Can you work these out from the model? Positions are in its coordinate system, mm. A direction names the side the tool comes from. Give positions to 0.01 mm unless a question says otherwise; leave off trailing zeros. Write each loop counter-clockwise with the first axis right and the second up, starting at its lowest first coordinate (ties: lowest second). Pieces come first, ordered by that corner, then holes.
1. Suppose I cut it at C-C (x = 5). Please give me the cut outline in (y, z), and give its area (3 significant figures).
2. Thinking about a two-plate mould opening in X: for faces 4 (the flat face through (48, -17.145, 3)), 5 (the cylindrical face through (-1.1, -74.92, 2.66)), 6 (the cylindrical face through (7.704, -24.063, 2.661)), which applies, pulls with the +X half, pulls with the -X half, needs draft (parallel to the pull), parting line crosses it, or undercut?
3. Suppose I cut it at D-D (y = -25.4). Give the number of separate pieces and of enclosed holes in the cut face, and give its area (3 significant figures).
4. Suppose I cut it at B-B (x = -46.99). Please give me the cut outline in (y, z) (1 decimal), and give its area (3 significant figures).
5. On a 3-axis mill with a long thin cutter (end or side, diameter ignored), from which of +Z, -Z, +X, -X, +Y, -Y can I reach the whole of each face in a straight line? I mean faces 1 (the cylindrical face through (0.41, -22.25, 2.74)), 2 (the cylindrical face through (-9.535, -20.621, 2.661)), 3 (the flat face through (54.55, -27, 3)). Say none if no direction works.
6. Suppose I cut it at A-A (y = -39.5). Please give me the cut outline in (x, z), and give its area (3 significant figures).
7. If I drill on probe 1 along X at (y, z) = (-28, 3.85); probe 2 along X at (y, z) = (-37.5, 1.35); probe 3 along X at (y, z) = (-39, 1.1), over which ranges is the centre line in solid material (lowest first)?
8. I'm going to push flat-ended pins straight in: pin 1 (5 mm diameter, centred on x = 0, y = -25.4, fed in from +Z); pin 2 (1.5 mm diameter, centred on x = 11.5, z = 2, fed in from +Y); pin 3 (1 mm diameter, centred on y = -51.5, z = 2, fed in from +X); pin 4 (1.6 mm diameter, centred on x = 34.5, z = 3, fed in from +Y) (3 decimals). Where does each tip first touch, or does it pass through?
```python
from build123d import *

# Parameters (mm, degrees)
SKETCH1_R                 = 1.651
BOSS_EXTRUDE2_DEPTH       = 5.3975
SKETCH2_R                 = 1.143
CUT_EXTRUDE1_DEPTH        = 6.3975
SKETCH3_R                 = 12.1285
CUT_EXTRUDE2_DEPTH        = 6.3975
SKETCH4_W                 = 28.562713242
SKETCH4_H                 = 11.677503754
BOSS_EXTRUDE3_DEPTH       = 5.3975
SKETCH5_W                 = 216.7214489
SKETCH5_H                 = 130.569220634
CUT_EXTRUDE4_DEPTH        = 6.3975
SKETCH7_R                 = 2
CUT_EXTRUDE5_DEPTH        = 23.368
SKETCH11_W                = 11.43
SKETCH11_H                = 10.16
CUT_EXTRUDE9_DEPTH        = 6.3975
SKETCH67_R                = 1.651
CUT_EXTRUDE65_DEPTH       = 97.79
SKETCH121_R               = 3.175
CUT_EXTRUDE119_DEPTH      = 103.378
CUT_EXTRUDE119_DEPTH_BACK = 48.768
CUT_EXTRUDE12_DEPTH       = 10
FILLET1_R                 = 2.54


with BuildPart() as part:
    # Sketch1 → Boss-Extrude2 (new body)
    with BuildSketch(Plane.XY):
        with BuildLine():
            Line((-64.964441474, 37.338), (-54.550441474, 37.338))
            Line((-54.550441474, 37.338), (-54.550441474, -37.338))
            Line((-54.550441474, -37.338), (-64.964441474, -37.338))
            ThreePointArc((-64.964441474, -37.338), (0, -74.93), (64.964441474, -37.338))
            Line((64.964441474, -37.338), (54.550441474, -37.338))
            Line((54.550441474, -37.338), (54.550441474, 37.338))
            Line((54.550441474, 37.338), (64.964441474, 37.338))
            ThreePointArc((64.964441474, 37.338), (0, 74.93), (-64.964441474, 37.338))
        make_face()
        with Locations((-46.482, 11.049)):
            Circle(SKETCH1_R, mode=Mode.SUBTRACT)
        with Locations((-21.083270032, 10.795)):
            Circle(SKETCH1_R, mode=Mode.SUBTRACT)
        with Locations((-21.083270032, -10.795)):
            Circle(SKETCH1_R, mode=Mode.SUBTRACT)
        with Locations((-46.482, -11.049)):
            Circle(SKETCH1_R, mode=Mode.SUBTRACT)
        with Locations((46.482, -11.049)):
            Circle(SKETCH1_R, mode=Mode.SUBTRACT)
        with Locations((21.083270032, -10.795)):
            Circle(SKETCH1_R, mode=Mode.SUBTRACT)
        with Locations((21.083270032, 10.795)):
            Circle(SKETCH1_R, mode=Mode.SUBTRACT)
        with Locations((46.482, 11.049)):
            Circle(SKETCH1_R, mode=Mode.SUBTRACT)
    extrude(amount=BOSS_EXTRUDE2_DEPTH)

    # Sketch2 → Cut-Extrude1 (cut, through all)
    with BuildSketch(Plane.XY.offset(5.3975)):
        with Locations((-6.731, 62.23)):
            Circle(SKETCH2_R)
        with Locations((6.731, 62.23)):
            Circle(SKETCH2_R)
    extrude(amount=-CUT_EXTRUDE1_DEPTH, mode=Mode.SUBTRACT)

    # Sketch3 → Cut-Extrude2 (cut, through all)
    with BuildSketch(Plane(origin=(0, 0, 0), x_dir=(-1, 0, 0), z_dir=(0, 0, -1))):
        with Locations((-43.105229381, -43.105229381)):
            Circle(SKETCH3_R)
        with Locations((14.224, -34.29)):
            Circle(SKETCH3_R)
        with Locations((14.224, 34.29)):
            Circle(SKETCH3_R)
        with Locations((-43.105229381, 43.105229381)):
            Circle(SKETCH3_R)
        with Locations((43.105229381, 43.105229381)):
            Circle(SKETCH3_R)
        with Locations((-14.224, 34.29)):
            Circle(SKETCH3_R)
        with Locations((-14.224, -34.29)):
            Circle(SKETCH3_R)
        with Locations((43.105229381, -43.105229381)):
            Circle(SKETCH3_R)
    extrude(amount=-CUT_EXTRUDE2_DEPTH, mode=Mode.SUBTRACT)

    # Sketch4 → Boss-Extrude3 (add)
    with BuildSketch(Plane(origin=(0, 0, 0), x_dir=(-1, 0, 0), z_dir=(0, 0, -1))):
        with Locations((-1.488809975, 62.152540216)):
            Rectangle(SKETCH4_W, SKETCH4_H)
    extrude(amount=-BOSS_EXTRUDE3_DEPTH)

    # Sketch5 → Cut-Extrude4 (cut, through all)
    with BuildSketch(Plane(origin=(0, 0, 0), x_dir=(-1, 0, 0), z_dir=(0, 0, -1))):
        with Locations((23.316688373, 48.139610317)):
            Rectangle(SKETCH5_W, SKETCH5_H)
    extrude(amount=-CUT_EXTRUDE4_DEPTH, mode=Mode.SUBTRACT)

    # Sketch7 → Cut-Extrude5 (cut)
    with BuildSketch(Plane(origin=(0, 0, 0), x_dir=(-1, 0, 0), z_dir=(0, 0, -1))):
        with Locations((0, -57.145)):
            Circle(SKETCH7_R)
    extrude(amount=-CUT_EXTRUDE5_DEPTH, mode=Mode.SUBTRACT)

    # Sketch11 → Cut-Extrude9 (cut, through all)
    with BuildSketch(Plane(origin=(0, 0, 0), x_dir=(-1, 0, 0), z_dir=(0, 0, -1))):
        with Locations((-33.595441474, -22.225)):
            Rectangle(SKETCH11_W, SKETCH11_H)
        with Locations((33.595441474, -22.225)):
            Rectangle(SKETCH11_W, SKETCH11_H)
    extrude(amount=-CUT_EXTRUDE9_DEPTH, mode=Mode.SUBTRACT)

    # Sketch67 → Cut-Extrude65 (cut)
    with BuildSketch(Plane(origin=(30.092005081, 4.08352975, -19.2405), x_dir=(-1, 0, 0), z_dir=(0, 0, -1))):
        with Locations((4.154396091, -49.728759131)):
            Circle(SKETCH67_R)
        with Locations((56.02961407, -49.728759131)):
            Circle(SKETCH67_R)
    extrude(amount=-CUT_EXTRUDE65_DEPTH, mode=Mode.SUBTRACT)

    # Sketch121 → Cut-Extrude119 (cut, two sides)
    with BuildSketch(Plane(origin=(30.092005081, 4.08352975, 16.891), x_dir=(-1, 0, 0), z_dir=(0, 0, -1))) as cut_extrude119_sk:
        with Locations((77.082005081, -29.48352975)):
            Circle(SKETCH121_R)
        with Locations((30.092005081, -29.48352975)):
            Circle(SKETCH121_R)
        with Locations((-16.897994919, -29.48352975)):
            Circle(SKETCH121_R)
    extrude(amount=CUT_EXTRUDE119_DEPTH, mode=Mode.SUBTRACT)
    extrude(cut_extrude119_sk.sketch, amount=-CUT_EXTRUDE119_DEPTH_BACK, mode=Mode.SUBTRACT)

    # Sketch14 → Cut-Extrude12 (cut)
    with BuildSketch(Plane.XY.offset(5.3975)):
        with BuildLine():
            Line((12.7, -20.24), (8.888991966, -20.24))
            ThreePointArc((8.888991966, -20.24), (5.715, -23.495), (2.541008034, -20.24))
            Line((2.541008034, -20.24), (-2.541008034, -20.24))
            ThreePointArc((-2.541008034, -20.24), (-5.715, -23.495), (-8.888991966, -20.24))
            Line((-8.888991966, -20.24), (-12.7, -20.24))
            ThreePointArc((-12.7, -20.24), (-16.235533906, -11.704466094), (-7.7, -15.24))
            Line((-7.7, -15.24), (7.7, -15.24))
            ThreePointArc((7.7, -15.24), (16.235533906, -11.704466094), (12.7, -20.24))
        make_face()
    extrude(amount=-CUT_EXTRUDE12_DEPTH, mode=Mode.SUBTRACT)

    # Fillet1
    fillet1_edges = [part.edges().sort_by_distance(p)[0] for p in [
        (39.310441474, -17.145, 2.69875),
        (27.880441474, -17.145, 2.69875),
        (-27.880441474, -17.145, 2.69875),
        (-39.310441474, -17.145, 2.69875),
        (-2.541008034, -20.24, 2.69875),
        (-8.888991966, -20.24, 2.69875),
        (-17.322875188, -17.145, 2.69875),
        (17.322875188, -17.145, 2.69875),
        (8.888991966, -20.24, 2.69875),
        (2.541008034, -20.24, 2.69875),
    ]]
    fillet(fillet1_edges, radius=FILLET1_R)


solid = part.part
```
Checks:
1. outline: (-74.76, 0) - (-42.17, 0) - (-42.17, 5.4) - (-74.76, 5.4) - close; (-26.41, 0) - (-23.41, 0) - (-23.41, 5.4) - (-26.41, 5.4) - close
1. area: 192 mm2
2. face 4: needs draft
2. face 5: parting line crosses it
2. face 6: undercut
3. separate pieces: 8
3. enclosed holes: 0
3. area: 185 mm2
4. outline: (-58.4, 0) - (-54.6, 0) - (-54.6, 5.4) - (-58.4, 5.4) - close; (-31.6, 0) - (-28.6, 0) - (-28.6, 5.4) - (-31.6, 5.4) - close; (-22.2, 0) - (-17.1, 0) - (-17.1, 5.4) - (-22.2, 5.4) - close
4. area: 64.2 mm2
5. face 1: +Z, -Z
5. face 2: +Z, -Z, +Y
5. face 3: +Z, -Z, +X, +Y
6. outline: (-63.67, 0) - (-54.69, 0) - (-54.69, 5.4) - (-63.67, 5.4) - close; (-31.52, 0) - (-25.18, 0) - (-25.18, 5.4) - (-31.52, 5.4) - close; (-3.27, 0) - (3.27, 0) - (3.27, 5.4) - (-3.27, 5.4) - close; (25.18, 0) - (31.52, 0) - (31.52, 5.4) - (25.18, 5.4) - close; (54.69, 0) - (63.67, 0) - (63.67, 5.4) - (54.69, 5.4) - close
6. area: 201 mm2
7. probe 1: x = -54.55 to -48.81, -45.17 to -24.59, -3.85 to -1.82, 1.82 to 3.85, 24.59 to 45.17, 48.81 to 54.55
7. probe 2: x = -64.87 to -53.86, -32.35 to -25.92, -2.53 to 2.53, 25.92 to 32.35, 53.86 to 64.87
7. probe 3: x = -63.98 to -54.52, -31.69 to -25.4, -3.05 to 3.05, 25.4 to 31.69, 54.52 to 63.98
8. pin 1: passes through
8. pin 2: stops at y = -20.24
8. pin 3: stops at x = 54.9
8. pin 4: stops at y = -27.305
